from build123d import *

# Parameters (mm, degrees)
SKETCH_1_W      = 30
SKETCH_1_H      = 25
EXTRUDE_2_DEPTH = 6
FILLET_2_R      = 2


with BuildPart() as part:
    # 스케치1 → 보스-돌출2 (new body)
    with BuildSketch(Plane.XY):
        Rectangle(SKETCH_1_W, SKETCH_1_H)
        with BuildLine():
            ThreePointArc((-5, -3.5), (-8.5, 0), (-5, 3.5))
            Line((-5, 3.5), (5, 3.5))
            ThreePointArc((5, 3.5), (7.474873734, 2.474873734), (8.5, 0))
            ThreePointArc((8.5, 0), (7.474873734, -2.474873734), (5, -3.5))
            Line((5, -3.5), (-5, -3.5))
        make_face(mode=Mode.SUBTRACT)
    extrude(amount=EXTRUDE_2_DEPTH)

    # 필렛2
    fillet_2_edges = [part.edges().sort_by_distance(p)[0] for p in [
        (-15, -12.5, 3),
        (-15, 12.5, 3),
        (15, 12.5, 3),
        (15, -12.5, 3),
    ]]
    fillet(fillet_2_edges, radius=FILLET_2_R)


solid = part.part
Check sheet for the modelled part. Datum: model origin and axes. Units: mm. A direction names the side the tool comes from. Give positions to 0.01 mm unless a question says otherwise; leave off trailing zeros. Write each loop counter-clockwise with the first axis right and the second up, starting at its lowest first coordinate (ties: lowest second). Pieces come first, ordered by that corner, then holes. Notation, with made-up numbers: (-31.5, 8.5) -> (21.5, 8.5) arc R34 cw to (21.5, 39.5) -> close; hole circle Ø10 at (12.5, 70.5). An arc over 180 degrees is marked (long way). One line per item, written item: value. Start each with the question number.
Item 1: Section check B-B on y = -2.5. Record the cut outline in (x, z), then the cut area to 3 significant figures.
Item 2: Gauge pin test, flat end, axial feed: pin 1 (5 mm diameter, centred on x = 2.5, y = -9, fed in from -Z). Record the tip position at first contact, or that the pin passes through.
Item 3: Draft check along Y on faces 1 (the cylindrical face through (14.4, 11.93, 3.04)), 2 (the flat face through (0, 3.5, 3)), 3 (the flat face through (0, 6, 0)). Enter one of: +Y half, -Y half, draft (parallel to the pull), parting line (faces both ways), or undercut.
Item 4: Section check A-A on z = 1.3. Record the cut outline in (x, y), then the cut area to 3 significant figures.
Item 5: Material ranges on probe 1 along Y at (x, z) = (1.25, 1.8); probe 2 along Y at (x, z) = (-7.5, 1.55); probe 3 along X at (y, z) = (-1, 5), recorded low to high. Write a range as from..to.
Item 6: Tool access check on faces 4 (the cylindrical face through (-8.5, -0.1, 3)), 5 (the flat face through (0, 6, 6)). Record the directions out of +Z, -Z, +X, -X, +Y, -Y that give a thin tool (end or side, any length) a straight path to the whole face; none if there is none.
Results list:
1. outline: (-15, 0) -> (-7.45, 0) -> (-7.45, 6) -> (-15, 6) -> close; (7.45, 0) -> (15, 0) -> (15, 6) -> (7.45, 6) -> close
1. area: 90.6 mm²
2. pin 1: z = 0
3. face 1: +Y half
3. face 2: undercut
3. face 3: draft
4. outline: (-15, -10.5) arc R2 ccw to (-13, -12.5) -> (13, -12.5) arc R2 ccw to (15, -10.5) -> (15, 10.5) arc R2 ccw to (13, 12.5) -> (-13, 12.5) arc R2 ccw to (-15, 10.5) -> close; hole (-5, -3.5) -> (5, -3.5) arc R3.5 ccw to (5, 3.5) -> (-5, 3.5) arc R3.5 ccw to start
4. area: 638 mm²
5. probe 1: -12.5..-3.5, 3.5..12.5
5. probe 2: -12.5..-2.45, 2.45..12.5
5. probe 3: -15..-8.35, 8.35..15
6. face 4: +Z, -Z
6. face 5: +Z, +X, -X, +Y, -Y
